from build123d import *

# Parameters (mm, degrees)
F4_DEPTH = 1
F3_W     = 12.4513199553
F3_H     = 2.5294316001
F5_W     = 74.8214920866
F5_H     = 12.595169118
F6_DEPTH = 0.01
F7_SCALE = 0.5


with BuildPart() as f4:
    # F3 (on Top) → F4 (new body)
    with BuildSketch(Plane.XY):
        with BuildLine():
            Line((-32.5062275336, -7.6), (-29.4775575647, -7.6))
            Line((-29.4775575647, -7.6), (-29.4327614695, -2.6532297294))
            Line((-29.4327614695, -2.6532297294), (-24.8831383838, -2.6532297294))
            Line((-24.8831383838, -2.6532297294), (-22.0433248124, -7.6))
            Line((-22.0433248124, -7.6), (-18.9124204973, -7.6))
            Line((-18.9124204973, -7.6), (-21.7522340687, -2.6532297294))
            ThreePointArc((-21.7522340687, -2.6532297294), (-20.2830658587, -2.0796278446), (-19.4100086076, -0.7661418768))
            Line((-19.4100086076, -0.7661418768), (-19.4100086076, 3.1799558435))
            ThreePointArc((-19.4100086076, 3.1799558435), (-20.1465672733, 4.3424852653), (-21.3581765803, 4.995169118))
            Line((-21.3581765803, 4.995169118), (-32.4662169309, 4.995169118))
            Line((-32.4662169309, 4.995169118), (-32.4662169309, 2.3768300461))
            Line((-32.4662169309, 2.3768300461), (-22.156490013, 2.3768300461))
            Line((-22.156490013, 2.3768300461), (-22.156490013, 0))
            Line((-22.156490013, 0), (-32.5062275336, 0))
            Line((-32.5062275336, 0), (-32.5062275336, -7.6))
        make_face()
    extrude(amount=F4_DEPTH)



with BuildPart() as f4b:
    # F3 (on Top) → F4, piece 2 (new body)
    with BuildSketch(Plane.XY):
        Polygon((-14.1395051198, 4.9199829809), (-17.3628383068, 4.9199829809), (-11.9944959487, -2.7468044573), (-11.9944959487, -7.6), (-9.3944959487, -7.6), (-9.3944959487, -2.7468044573), (-4.0261535905, 4.9199829809), (-7.2494867775, 4.9199829809), (-10.6944959487, 0), align=None)
    extrude(amount=F4_DEPTH)


with BuildPart() as f4c:
    # F3 (on Top) → F4, piece 3 (new body)
    with BuildSketch(Plane.XY):
        Polygon((-1.5607364842, 4.8494239393), (-1.5607364842, 2.2384772427), (6.939469985, 2.2384772427), (-1.5920158667, -5.0374310329), (-1.5920158667, -7.6), (10.8593031573, -7.6), (10.8593031573, -5.0839300849), (2.4482466872, -5.0839300849), (11.0528468894, 2.399763919), (11.0528468894, 4.8494239393), align=None)
    extrude(amount=F4_DEPTH)


with BuildPart() as f4d:
    # F3 (on Top) → F4, piece 4 (new body)
    with BuildSketch(Plane.XY):
        with Locations((20.4074648017, 3.4706616363)):
            Rectangle(F3_W, F3_H)
    extrude(amount=F4_DEPTH)


with BuildPart() as f4e:
    # F3 (on Top) → F4, piece 5 (new body)
    with BuildSketch(Plane.XY):
        Polygon((14.0850310954, -7.6), (26.6331247794, -7.6), (26.6331247794, -5.1448669866), (16.9365629362, -5.1448669866), (16.9365629362, -2.5965400156), (26.6331247794, -2.5965400156), (26.6331247794, -0.1888843136), (14.0850310954, -0.1888843136), align=None)
    extrude(amount=F4_DEPTH)


with BuildPart() as f4f:
    # F3 (on Top) → F4, piece 6 (new body)
    with BuildSketch(Plane.XY):
        Polygon((29.911786692, -7.6), (32.6458275334, -7.6), (32.6458275334, 0.3624289589), (39.5166337506, -7.6), (42.3552751557, -7.6), (42.3552751557, 4.5534580069), (39.4317097559, 4.5534580069), (39.4317097559, -3.4268074825), (32.5400491226, 4.7125679496), (29.911786692, 4.7125679496), align=None)
    extrude(amount=F4_DEPTH)


with BuildPart() as f4_1:
    add(f4.part)

    add(f4b.part)  # F6 merges F4b

    add(f4c.part)  # F6 merges F4c

    add(f4d.part)  # F6 merges F4d

    add(f4e.part)  # F6 merges F4e

    add(f4f.part)  # F6 merges F4f
    # F5 (on Top) → F6 (join)
    with BuildSketch(Plane.XY):
        with Locations((4.9445291124, -1.302415441)):
            Rectangle(F5_W, F5_H)
    extrude(amount=-F6_DEPTH)


with BuildPart() as f4_2:
    # F7: moved
    add(f4_1.part.scale(F7_SCALE))


solid = f4_2.part
Input: part model. Units: mm. Frame: model coordinates. A direction names the side the tool comes from. Coordinates: 2 decimals unless noted, no trailing zeros. Loops run counter-clockwise (first coordinate to the right, second up) from the corner with the lowest first, then second, coordinate; pieces in that order, holes last.
(1) Set-up query: faces 1 (the face through (-3.37, 0.52, 0.25)), 2 (the face through (-4.47, 1.25, 0.25)), 3 (the face through (2, -1, -0.005)), 4 (the face through (1.37, -0.67, 0.25)). Return all of +Z, -Z, +X, -X, +Y, -Y with unobstructed straight access to the full face (end or side cutting, diameter ignored); none if empty.
(2) Pull-direction query (X, two-part tool) for faces 5 (the face through (18, -1, 0.5)), 6 (the face through (3.345, -0.697, 0.246)); classes: released by +X, released by -X, zero draft, split by the parting line, or undercut.
(3) Section D-D on x = -12. Return the cut outline in (y, z) (3 decimals).
(4) Material intervals for probe 1 along Y at (x, z) = (11.5, 0.35); probe 2 along Y at (x, z) = (2, 0.1); probe 3 along Y at (x, z) = (-13, 0.2), sorted ascending.
(5) Section A-A on x = 15.5. Return the cut outline in (y, z) (3 decimals), then the cut area to 3 significant figures.
(6) Section B-B on z = 0.4. Count the separate pieces of the cut face and the enclosed holes in it, then the cut area to 3 significant figures.
Data:
1. face 1: +Z, -Y
1. face 2: +Z, +Y
1. face 3: -Z, +X, -X, +Y, -Y
1. face 4: +Z
2. face 5: zero draft
2. face 6: undercut
3. outline: (-3.8, -0.005) - (2.498, -0.005) - (2.498, 0.5) - (1.188, 0.5) - (1.188, 0) - (0, 0) - (0, 0.5) - (-2.096, 0.5) - (-2.096, 0) - (-3.8, 0) - close
4. probe 1: y = -3.8 to -2.57, -1.3 to -0.09, 1.1 to 2.37
4. probe 2: y = -3.8 to -2.54, -1.87 to -0.13, 1.12 to 2.42
4. probe 3: y = -1.33 to 0, 1.19 to 2.5
5. outline: (-3.8, -0.005) - (2.498, -0.005) - (2.498, 0) - (2.356, 0) - (2.356, 0.5) - (-3.8, 0.5) - close
5. area: 3.11 mm2
6. separate pieces: 6
6. enclosed holes: 0
6. area: 113 mm2
